For this review, use the dimensioned drawing (mm, ordinates from the lowest corner) and the shaded views. A direction names the side the tool comes from. Give positions to 0.01 mm unless a question says otherwise; leave off trailing zeros. Loops run counter-clockwise (first coordinate to the right, second up) from the corner with the lowest first, then second, coordinate; pieces in that order, holes last. Notation, with made-up numbers: M 75,44.25 L 89,44.25 A18 ccw 89,48.25 Z; hole C 85.5,0 d3. An arc over 180 degrees is marked long. Use CSV: the item, a comma, the result in double quotes.
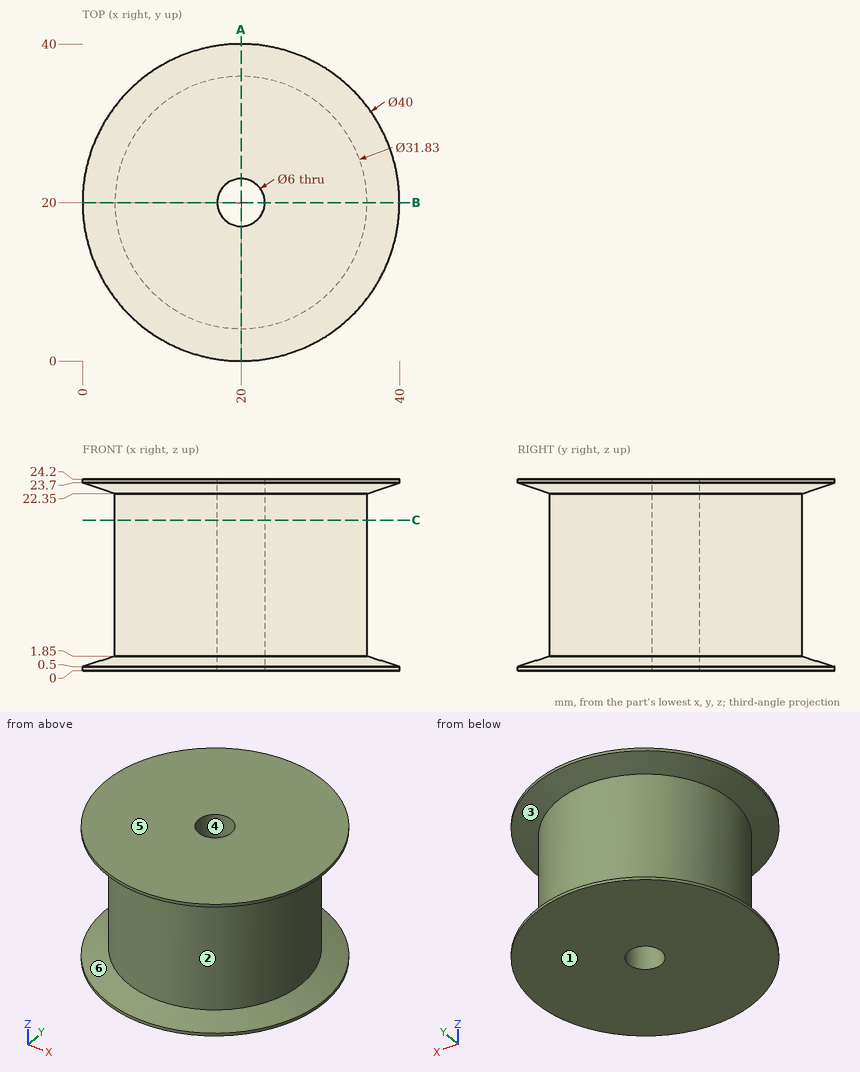
(1) Wall thickness on line 1 along Y through (x, z) = (20, 18.25) (3 decimals); line 2 along Z through (x, y) = (33.5, 28.5); line 3 along Y through (x, z) = (17.5, 7.25): over which ranges is each line inside the solid? List them lowest first. Write a range as [from, to].
A:
line 1,"[4.085, 17], [23, 35.915]"
line 2,"[0, 1.84], [22.36, 24.2]"
line 3,"[4.28, 18.34], [21.66, 35.72]"
(2) Clearance check with flat-ended pins moving along their axes: P1, Ø10, axis at x = 36, z = 15, coming from the +Y side; P2, Ø2, axis at y = 17.5, z = 19, coming from the +X side; P3, Ø12, axis at x = 14, z = 19.5, coming from the -Y side. State where each tip first meets the part, or that it passes through.
A:
P1,"y = 31.5"
P2,"x = 35.84"
P3,"y = 0.07"
(3) The part is to be moulded in two halves that separate along Z. For the marked faces 1, 2, 3 and 4, say which applies: released by +Z, released by -Z, zero draft, split by the parting line, or undercut.
A:
face 1,"released by -Z"
face 2,"undercut"
face 3,"undercut"
face 4,"zero draft"
(4) Machinability: for the marked faces 5 and 6, which of the approach directions +Z, -Z, +X, -X, +Y, -Y give a long, thin tool a straight path to every point of the face, cutting with its end or side? Answer none if there is none.
A:
face 5,"+Z, +X, -X, +Y, -Y"
face 6,"none"
(5) We need section C-C on z = 19. State the section outline as (x, y) points (3 decimals).
A:
outline,"C 20,20 d31.83; hole C 20,20 d6"
(6) We need section A-A on x = 20. State the section outline as (y, z) points (3 decimals).
A:
outline,"M 0,0 L 17,0 L 17,24.2 L 0,24.2 L 0,23.7 L 4.085,22.35 L 4.085,1.85 L 0,0.5 Z; M 23,0 L 40,0 L 40,0.5 L 35.915,1.85 L 35.915,22.35 L 40,23.7 L 40,24.2 L 23,24.2 Z"
